Design review of the part built by this model. Coordinates are the model's own, in mm. Face numbers are marked on the shaded views. A direction names the side the tool comes from. Round coordinates to 2 decimals unless told otherwise and drop trailing zeros. Loops run counter-clockwise (first coordinate to the right, second up) from the corner with the lowest first, then second, coordinate; pieces in that order, holes last. Notation, with made-up numbers: M -30,16 L 25,16 A20 cw 25,26 Z; hole C 25.5,56.5 d11. An arc over 180 degrees is marked long. One line per item, written item: value. Start each with the question number.
Item 1: Clearance check with flat-ended pins moving along their axes: pin 1 (3 mm diameter, centred on x = 1, y = 4, fed in from -Z); pin 2 (2 mm diameter, centred on x = 10, y = 1.5, fed in from +Z); pin 3 (4 mm diameter, centred on x = -1, z = 26.5, fed in from +Y); pin 4 (3 mm diameter, centred on x = -2, y = 3, fed in from +Z). State where each tip first meets the part, or that it passes through.
Item 2: We need section A-A (z = 9). Write out the cut boundary in (x, y), then the cut area to 3 significant figures.
Item 3: Mouldability with a two-part tool opening along Z and no side actions: class the marked faces 1, 2 and 3 as released by +Z, released by -Z, zero draft, split by the parting line, or undercut.
Item 4: For the marked faces 4 and 5, list the 3-axis set-ups (+Z, -Z, +X, -X, +Y, -Y) from which the entire face can be reached by the end or side of a thin tool; tool diameter is ignored.
Item 5: We need section C-C (x = -0.5). Write out the cut boundary in (y, z), then the cut area to 3 significant figures.
Item 6: For line 1 along Z through (x, y) = (0, 0.85); line 2 along X through (y, z) = (2.7, 9); line 3 along Z through (x, y) = (9, 2.05), list the stretches that pass through material, from the lowest coordinate up.
Item 7: We need section B-B (y = 2.9). Write out the cut boundary in (x, z), then the cut area to 3 significant figures.
Item 8: We need section D-D (x = 8). Write out the cut boundary in (y, z).
Autodesk Inventor part; units mm, degrees
ref_plane "YZ Plane" through (0, 0, 0) normal (1, 0, 0) x (0, 1, 0)
ref_plane "XZ Plane" through (0, 0, 0) normal (0, 1, 0) x (-1, 0, 0)
ref_plane "XY Plane" through (0, 0, 0) normal (0, 0, 1) x (1, 0, 0)
sketch "Sketch1" plane through (0, 0, 0) normal (0, 1, 0) x (-1, 0, 0)
  line L0 (0, 26) -> (0, 0)
  line L1 (0, 9) -> (6, 9)
  line L2 (6, 9) -> (-9, 9)
  line L3 (11, 6) -> (11, 16)
  line L4 (-14, 16) -> (-14, 6)
  line L5 (1, 30) -> (-1, 30)
  line L6 (-1, -4) -> (1, -4)
  arc A0 (5, 26) -> (1, 30) centre (1, 26) ccw
  arc A1 (-1, 30) -> (-5, 26) centre (-1, 26) ccw
  arc A2 (1, -4) -> (5, 0) centre (1, 0) ccw
  arc A3 (-5, 0) -> (-1, -4) centre (-1, 0) ccw
  line L7 (7, 22) -> (9, 22)
  line L8 (9, 4) -> (7, 4)
  line L9 (-12, 4) -> (-7, 4)
  line L10 (-7, 22) -> (-12, 22)
  line L11 (-14, 20) -> (-14, 16)
  line L12 (-5, 24) -> (-5, 26)
  line L13 (-5, 2) -> (-5, 0)
  arc A4 (-7, 22) -> (-5, 24) centre (-7, 24) ccw
  arc A5 (-12, 22) -> (-14, 20) centre (-12, 20) ccw
  arc A6 (-14, 6) -> (-12, 4) centre (-12, 6) ccw
  arc A7 (-5, 2) -> (-7, 4) centre (-7, 2) ccw
  line L14 (5, 26) -> (5, 24)
  line L15 (5, 2) -> (5, 0)
  arc A8 (5, 24) -> (7, 22) centre (7, 24) ccw
  arc A9 (11, 20) -> (9, 22) centre (9, 20) ccw
  arc A10 (9, 4) -> (11, 6) centre (9, 6) ccw
  arc A11 (7, 4) -> (5, 2) centre (7, 2) ccw
  line L16 (11, 16) -> (11, 20)
  line L17 (11, 16) -> (-14, 16)
  line L18 (9, 4) -> (-12, 4)
  circle A12 centre (6, 9) radius 1.5
  point P0 (0, 0)
  point P1 (-14, 4)
  point P2 (5, 22)
  point P3 (11, 22)
  point P4 (5, 4)
  dimension "d9" = 6
  dimension "d10" = 26
  dimension "d11" = 9
  dimension "d12" = 15
  dimension "d13" = 5
  dimension "d14" = 5
  dimension "d17" = 4
  dimension "d18" = 4
  dimension "d20" = 4
  dimension "d21" = 4
  dimension "d22" = 4
  dimension "d23" = 4
  dimension "d25" = 5
  dimension "d26" = 5
  dimension "d27" = 18
  dimension "d28" = 1
  dimension "d29" = 2
  dimension "d30" = 6
  dimension "d31" = 1
  dimension "d32" = 6
  dimension "d34" = 4
  dimension "d35" = 2
  dimension "d37" = 10
  dimension "d38" = 6
  dimension "d39" = 2
  dimension "d54" = 3
extrude "Extrusion1" add sketch "Sketch1" along normal blind 2 contours A12 | L17 L3 A10 L8 L18 L0 | L17 L11 A5 L10 A4 L12 A1 L5 A0 L14 A8 L7 A9 L16 | L0 L18 L9 A6 L4 L17 | L18 A11 L15 A2 L6 A3 L13 A7
extrude "Extrusion2" add sketch "Sketch1" along normal blind 4 contours A12 | L17 L3 A10 L8 L18 L0 | L0 L18 L9 A6 L4 L17
hole "Hole1" at (0, 0, 26) at (9, 0, 9) at (0, 0, 0) direction (0, 1, 0) diameter 3 depth 8 tip angle 118
extrude "Extrusion4" add sketch "Sketch1" along normal blind 5 contours A12
properties part number "imu_MPU6050Holder_V2"
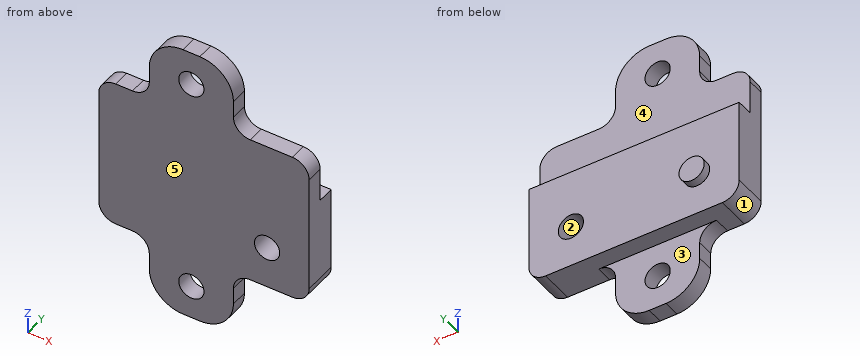
A:
1. pin 1: z = 4
1. pin 2: z = 22
1. pin 3: y = 2
1. pin 4: z = 30
2. outline: M -11,0 L 7.5,0 L 7.5,4 L -4.5,4 L -4.5,5 L -7.5,5 L -7.5,4 L -11,4 Z; M 10.5,0 L 14,0 L 14,4 L 10.5,4 Z
2. area: 91.0 mm2
3. face 1: released by -Z
3. face 2: undercut
3. face 3: zero draft
4. face 4: +Z, +X, -X, +Y
4. face 5: +Z, -Z, +X, -X, -Y
5. outline: M 0,-4 L 2,-4 L 2,-1.41 L 0,-1.41 Z; M 0,1.41 L 2,1.41 L 2,4 L 4,4 L 4,16 L 2,16 L 2,24.59 L 0,24.59 Z; M 0,27.41 L 2,27.41 L 2,30 L 0,30 Z
5. area: 80.7 mm2
6. line 1: -4 to -1.5, 1.5 to 24.5, 27.5 to 30
6. line 2: -11 to 7.5, 10.5 to 14
6. line 3: 4 to 7.5, 10.5 to 16
7. outline: M -11,6 A2 ccw -9,4 L 12,4 A2 ccw 14,6 L 14,16 L -11,16 Z; hole C 9,9 d3
7. area: 291 mm2
8. outline: M 0,4 L 4,4 L 4,7.88 L 0,7.88 Z; M 0,10.12 L 4,10.12 L 4,16 L 2,16 L 2,22 L 0,22 Z
